Can you work these out from the model? Positions are in its coordinate system, mm. Round coordinates to 2 decimals unless told otherwise and drop trailing zeros. Write each loop counter-clockwise with the first axis right and the second up, starting at its lowest first coordinate (ties: lowest second). Pieces come first, ordered by that corner, then holes.
Q1. Please list where these lines run through material, in increasing order: line 1 along X through (y, z) = (12, -16.5); line 2 along X through (y, z) = (3, -21.5); line 3 along Y through (x, z) = (12, -22).
Q2. If we section it at A-A (x = 13): Please give me the cut outline in (y, z), plus the area to 3 significant figures.
Q3. We'd pull the mould along Y, two halves only. Please class faces 1 (the flat face through (60, 20, -15)), 2 (the cylindrical face through (45.98, 22.43, -13.78)), 3 (the flat face through (30, 40, -15)): +Y half, -Y half, draft (parallel to the pull), parting line (faces both ways), or undercut.
Q4. If we section it at C-C (x = 32): Please give me the cut outline in (y, z).
Q5. If we section it at B-B (y = 9): Give the number of separate pieces and of enclosed holes in the cut face, plus the area to 3 significant figures.
from build123d import *

# Parameters (mm, degrees)
F0_W     = 60
F0_H     = 40
F1_DEPTH = 30
F2_SIZE  = 10
F4_D     = 9
F5_SIZE  = 1


with BuildPart() as f1:
    # F0 (on Top) → F1 (new body)
    with BuildSketch(Plane.XY):
        with Locations((30, 20)):
            Rectangle(F0_W, F0_H)
    extrude(amount=-F1_DEPTH)

    # F2
    f2_edges = [f1.edges().sort_by_distance(p)[0] for p in [
        (30, 0, -30),
    ]]
    chamfer(f2_edges, length=F2_SIZE)

    # F4 (through all)
    with Locations(Plane(origin=(0, -10, -10), x_dir=(1, 0, 0), z_dir=(0, -0.7071067812, -0.7071067812))):
        with Locations((15, -21.2132034356), (45, -21.2132034356)):
            Hole(F4_D / 2)

    # F5
    f5_edges = [f1.edges().sort_by_distance(p)[0] for p in [
        (30, 0, 0),
    ]]
    chamfer(f5_edges, length=F5_SIZE)


solid = f1.part
A:
1. line 1: x = 0 to 10.63, 19.37 to 40.63, 49.37 to 60
1. line 2: x = 0 to 12.74, 17.26 to 42.74, 47.26 to 60
1. line 3: y = 2 to 3.26, 12.74 to 40
2. outline: (0, -20) - (2.15, -22.15) - (24.3, 0) - (1, 0) - (0, -1) - close; (7.85, -27.85) - (10, -30) - (40, -30) - (40, 0) - (35.7, 0) - close
2. area: 864 mm2
3. face 1: draft
3. face 2: undercut
3. face 3: +Y half
4. outline: (0, -20) - (10, -30) - (40, -30) - (40, 0) - (1, 0) - (0, -1) - close
5. separate pieces: 1
5. enclosed holes: 2
5. area: 1,560 mm2
